from build123d import *

# Parameters (mm, degrees)
REVOLVE1_ANGLE = 60


with BuildPart() as part:
    # Sketch1 → Revolve1 (revolve)
    with BuildSketch(Plane.XY):
        with BuildLine():
            Line((-45, 1.936673673), (-10, 1.936673673))
            Line((-10, 1.936673673), (-10, 2.436673673))
            Line((-10, 2.436673673), (-45.000375853, 2.436673673))
            ThreePointArc((-45.000375853, 2.436673673), (-45.557674224, 2.435543108), (-46.114971099, 2.433826721))
            ThreePointArc((-46.114971099, 2.433826721), (-177.046295247, -14.475660779), (-299.740246695, -63.211034879))
            Line((-299.740246695, -63.211034879), (-299.499248826, -63.64912166))
            ThreePointArc((-299.499248826, -63.64912166), (-176.921010606, -14.959710114), (-46.11316839, 1.933829971))
            ThreePointArc((-46.11316839, 1.933829971), (-45.556584942, 1.935544259), (-45, 1.936673673))
        make_face()
    revolve(axis=Axis((0, -998.5, 0), (0, 1, 0)), revolution_arc=REVOLVE1_ANGLE)


solid = part.part
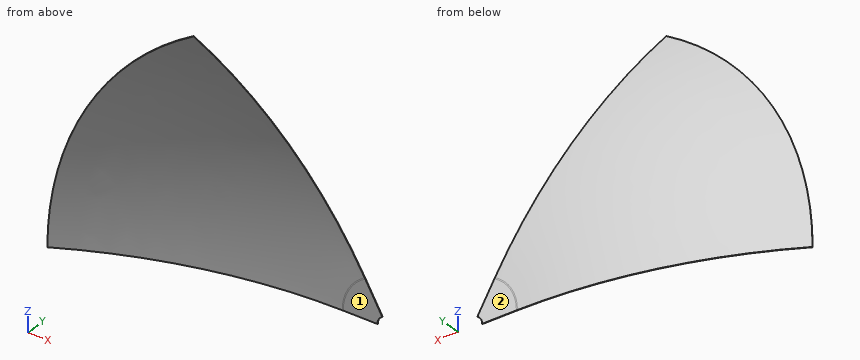
Geometry: final body of the model. Coordinates: model frame, mm. Face numbers are marked on the shaded views. A direction names the side the tool comes from. Round coordinates to 2 decimals unless told otherwise and drop trailing zeros.
Q1. Material intervals for L1, parallel to Y at x = -143, z = 45; L2, parallel to Y at x = -97.5, z = 124; L3, parallel to Z at x = -194, y = -60, sorted ascending.
Q2. Pin query (flat end, axial travel): P1, Ø1.5, axis at x = -123, z = 148, coming from the +Y side; P2, Ø19.5, axis at x = -24, z = 22.5, coming from the -Y side. Return the tip coordinate at first contact, or that it passes through.
Q3. Access query for the marked faces 1 and 2. Directions: +Z, -Z, +X, -X, +Y, -Y. A direction counts if a zero-diameter tool reaches every point of the face in a straight line with its end or side. Return the directions, or none.
Evaluation:
1. L1: y = -8.72 to -8.21
1. L2: y = -10.37 to -9.86
1. L3: z = 219.24 to 220.66
2. P1: stops at y = -18.49
2. P2: stops at y = 1.94
3. face 1: -Z, +X, -Y
3. face 2: +Z, -Z, +X, -X, +Y
